```python
from build123d import *

# Parameters (mm, degrees)
SKETCH_1_W          = 290
SKETCH_1_H          = 290
EXTRUDE_1_DEPTH     = 60
SKETCH_2_W          = 280
SKETCH_2_H          = 280
CUT_EXTRUDE_2_DEPTH = 55
SKETCH_3_W          = 224
SKETCH_3_H          = 138
CUT_EXTRUDE_3_DEPTH = 5
SKETCH_4_R          = 1.4
CUT_EXTRUDE_4_DEPTH = 5
FILLET_1_R          = 10
FILLET_2_R          = 10


with BuildPart() as part:
    # 草图1 → 凸台-拉伸1 (new body)
    with BuildSketch(Plane(origin=(0, 0, 0), x_dir=(1, 0, 0), z_dir=(0, 1, 0))):
        Rectangle(SKETCH_1_W, SKETCH_1_H)
    extrude(amount=EXTRUDE_1_DEPTH)

    # 草图2 → 切除-拉伸2 (cut)
    with BuildSketch(Plane(origin=(0, 60, 0), x_dir=(1, 0, 0), z_dir=(0, 1, 0))):
        Rectangle(SKETCH_2_W, SKETCH_2_H)
    extrude(amount=-CUT_EXTRUDE_2_DEPTH, mode=Mode.SUBTRACT)

    # 草图3 → 切除-拉伸3 (cut)
    with BuildSketch(Plane(origin=(0, 5, 0), x_dir=(1, 0, 0), z_dir=(0, 1, 0))):
        Rectangle(SKETCH_3_W, SKETCH_3_H)
    extrude(amount=-CUT_EXTRUDE_3_DEPTH, mode=Mode.SUBTRACT)

    # 草图4 → 切除-拉伸4 (cut)
    with BuildSketch(Plane.XZ):
        with Locations(Location((-122, 64, 0), (0, 0, 270))):
            Circle(SKETCH_4_R)
        with Locations(Location((122, 64, 0), (0, 0, 270))):
            Circle(SKETCH_4_R)
        with Locations(Location((122, -64, 0), (0, 0, 270))):
            Circle(SKETCH_4_R)
        with Locations(Location((-122, -64, 0), (0, 0, 270))):
            Circle(SKETCH_4_R)
    extrude(amount=-CUT_EXTRUDE_4_DEPTH, mode=Mode.SUBTRACT)

    # 圆角1
    fillet_1_edges = [part.edges().sort_by_distance(p)[0] for p in [
        (140, 32.5, -140),
        (-140, 32.5, -140),
        (-140, 32.5, 140),
        (140, 32.5, 140),
        (145, 30, 145),
        (-145, 30, 145),
        (-145, 30, -145),
        (145, 30, -145),
    ]]
    fillet(fillet_1_edges, radius=FILLET_1_R)

    # 圆角2
    fillet_2_edges = [part.edges().sort_by_distance(p)[0] for p in [
        (-112, 2.5, -69),
        (-112, 2.5, 69),
        (112, 2.5, 69),
        (112, 2.5, -69),
    ]]
    fillet(fillet_2_edges, radius=FILLET_2_R)


solid = part.part
```
Design review of the part built by this model. Coordinates are the model's own, in mm. A direction names the side the tool comes from. Give positions to 0.01 mm unless a question says otherwise; leave off trailing zeros. Order: outer loops, then holes, each group sorted by start corner. A loop starts at its lowest first (then second) coordinate and runs counter-clockwise, first axis right, second up. Notation, with made-up numbers: M 69.25,-36 L 113.25,-36 A26 cw 113.25,-2 Z; hole C -35,68 d1. An arc over 180 degrees is marked long. One line per question, with ' | ' between items. Start each with the question number.
Q1. For pin 1 Ø1.7 at (x, z) = (-122, 64) entering from +Y (3 decimals); pin 2 Ø10 at (x, z) = (-7, 112.5) entering from +Y, all flat-tipped, find the tip position at first contact; note any pin that passes through.
Q2. For L1, parallel to Z at x = 56, y = 29.5; L2, parallel to Z at x = -122, y = 2.55, list the stretches that pass through material, from the lowest coordinate up. Write a range as [from, to].
Q3. We need section A-A (x = -22). Write out the cut boundary in (y, z), plus the area to 3 significant figures.
Q4. We need section D-D (x = -117). Write out the cut boundary in (y, z), plus the area to 3 significant figures.
Q5. Machinability: for faces 4 (the face through (-2, 33, 140)), 5 (the face through (-108.99, 2.46, 66.15)), 6 (the face through (-2, 30, 145)), which of the approach directions +Z, -Z, +X, -X, +Y, -Y give a long, thin tool a straight path to every point of the face, cutting with its end or side? Answer none if there is none.
Q6. We need section C-C (y = 35). Write out the cut boundary in (x, z), plus the area to 3 significant figures.
Q7. The part is to be moulded in two halves that separate along Z. For faces 1 (the face through (-145, 30, 2)), 2 (the face through (-2, 30, -145)), 3 (the face through (108.99, 2.46, 66.15)), say which applies: +Z half, -Z half, draft (parallel to the pull), parting line (faces both ways), or undercut.
Q8. We need section B-B (z = -42). Write out the cut boundary in (x, y).
Returned:
1) pin 1: through | pin 2: y = 5
2) L1: [-145, -140], [140, 145] | L2: [-145, -65.4], [-62.6, 62.6], [65.4, 145]
3) outline: M 0,-145 L 60,-145 L 60,-140 L 5,-140 L 5,-69 L 0,-69 Z; M 0,69 L 5,69 L 5,140 L 60,140 L 60,145 L 0,145 Z | area: 1,310 mm2
4) outline: M 0,-145 L 60,-145 L 60,-140 L 5,-140 L 5,140 L 60,140 L 60,145 L 0,145 Z | area: 2,000 mm2
5) face 4: +Y | face 5: +Y, -Y | face 6: +Z, +X, -X, +Y, -Y
6) outline: M -145,-135 A10 ccw -135,-145 L 135,-145 A10 ccw 145,-135 L 145,135 A10 ccw 135,145 L -135,145 A10 ccw -145,135 Z; hole M -140,-130 A10 ccw -130,-140 L 130,-140 A10 ccw 140,-130 L 140,130 A10 ccw 130,140 L -130,140 A10 ccw -140,130 Z | area: 5,700 mm2
7) face 1: draft | face 2: -Z half | face 3: undercut
8) outline: M -145,0 L -112,0 L -112,5 L -140,5 L -140,60 L -145,60 Z; M 112,0 L 145,0 L 145,60 L 140,60 L 140,5 L 112,5 Z
